The listing builds one solid part. Answer for the finished solid, in the listing's coordinates (mm). A direction names the side the tool comes from. Round coordinates to 2 decimals unless told otherwise and drop trailing zeros. Order: outer loops, then holes, each group sorted by start corner. A loop starts at its lowest first (then second) coordinate and runs counter-clockwise, first axis right, second up. Notation, with made-up numbers: (29.5, 27.25) - (49.5, 27.25) arc R16 ccw to (49.5, 57.25) - close; hole circle Ø9 at (3.25, 59). An arc over 180 degrees is marked (long way). One line per item, written item: value. Start each with the question number.
1. Section D-D, the plane y = 9 is taken. Give the vertices of the cut face in (x, z).
2. Flat-ended cylindrical pins translate along their axes: P1, Ø1, axis at x = 4.5, y = 1.5, coming from the -Z side; P2, Ø5, axis at y = 4.5, z = 3.5, coming from the -X side; P3, Ø1.8, axis at x = 3, y = -5, coming from the -Z side; P4, Ø0.9, axis at x = 4, z = 1.5, coming from the -Y side. Find the tip coordinate at first contact, or state that the pin passes through.
3. Section C-C, the plane x = 3.9 is taken. Give the vertices of the cut face in (y, z), then the cut area to 3 significant figures.
4. For a pull along Y with two mould halves and no side action, classify faces 1 (the flat face through (3, 33, 1)), 2 (the flat face through (2.96, -7.21, 6.43)), 3 (the flat face through (3, 30, 2)), 4 (the flat face through (3, 0, 2)) as released by +Y, released by -Y, zero draft, split by the parting line, or undercut.
5. Section A-A, the plane z = 1 is taken. Give the vertices of the cut face in (x, y).
6. Section B-B, the plane z = 3.5 is taken. Give the vertices of the cut face in (x, y), then the cut area to 3 significant figures.
7. A tool of negligible diameter and unlimited length cuts with its end or side. For faces 5 (the cylindrical face through (2.958, 29.699, 4.715)), 6 (the flat face through (3, -6, 3)), 7 (the flat face through (3, 31, 0)), 8 (the flat face through (3, 36, 3)), 9 (the flat face through (3, -9, 4)), from which of +Z, -Z, +X, -X, +Y, -Y can it reach the whole face along a straight path? Write none if from no direction.
8. Straight lines are drawn through the part: line 1 (Y direction, x = 1.3, z = 3.5); line 2 (Y direction, x = 2.1, z = 1); line 3 (Z direction, x = 5.75, y = 20). For each, find the intervals that lie inside material, in ascending order.
Autodesk Inventor part; units mm, degrees
ref_plane "YZ Plane" through (0, 0, 0) normal (1, 0, 0) x (0, 1, 0)
ref_plane "XZ Plane" through (0, 0, 0) normal (0, 1, 0) x (-1, 0, 0)
ref_plane "XY Plane" through (0, 0, 0) normal (0, 0, 1) x (1, 0, 0)
sketch "Sketch1" plane through (0, 0, 0) normal (1, 0, 0) x (0, 1, 0)
  line L0 (30, 0) -> (33, 0)
  line L1 (33, 0) -> (33, 3)
  line L2 (33, 3) -> (39, 3)
  line L3 (-9, 3) -> (-3, 3)
  line L4 (-3, 3) -> (-3, 0)
  line L5 (-3, 0) -> (0, 0)
  line L6 (0, 0) -> (0, 4)
  line L7 (1, 5) -> (29, 5)
  line L8 (30, 4) -> (30, 0)
  arc A0 (1, 5) -> (0, 4) centre (1, 4) ccw
  arc A1 (30, 4) -> (29, 5) centre (29, 4) ccw
  line L9 (-4, 9) -> (34, 9)
  line L10 (34, 9) -> (39, 5)
  line L11 (39, 5) -> (39, 3)
  line L12 (-9, 3) -> (-9, 5)
  line L13 (-9, 5) -> (-4, 9)
  point P0 (0, 0)
  point P1 (0, 5)
  point P2 (30, 5)
  point P3 (15, 9)
  point P4 (15, 5)
  dimension "d1" = 3
  dimension "d4" = 30
  dimension "d5" = 2
  dimension "d7" = 3
  dimension "d30" = 38
  dimension "d31" = 4
  dimension "d32" = 2
  dimension "d33" = 2
  dimension "d36" = 3
  dimension "d37" = 3
  dimension "d41" = 6
  dimension "d42" = 6
extrude "Extrusion1" add sketch "Sketch1" along normal blind 6
fillet "Fillet1" radius 5 2 edges at (3, -4, 9) (3, 34, 9)
properties part number "27080914ServoMount"
Answer list:
1. outline: (0, 5) - (6, 5) - (6, 9) - (0, 9) - close
2. P1: stops at z = 5
2. P2: stops at x = 0
2. P3: stops at z = 3
2. P4: stops at y = -3
3. outline: (-9, 3) - (-3, 3) - (-3, 0) - (0, 0) - (0, 4) arc R1 cw to (1, 5) - (29, 5) arc R1 cw to (30, 4) - (30, 0) - (33, 0) - (33, 3) - (39, 3) - (39, 5) - (35.37, 7.9) arc R5 ccw to (32.25, 9) - (-2.25, 9) arc R5 ccw to (-5.37, 7.9) - (-9, 5) - close
3. area: 226 mm²
4. face 1: released by +Y
4. face 2: released by -Y
4. face 3: undercut
4. face 4: undercut
5. outline: (0, -3) - (6, -3) - (6, 0) - (0, 0) - close; (0, 30) - (6, 30) - (6, 33) - (0, 33) - close
6. outline: (0, -9) - (6, -9) - (6, 0) - (0, 0) - close; (0, 30) - (6, 30) - (6, 39) - (0, 39) - close
6. area: 108 mm²
7. face 5: -Z, +X, -X
7. face 6: -Z, +X, -X, -Y
7. face 7: -Z, +X, -X, +Y, -Y
7. face 8: -Z, +X, -X, +Y
7. face 9: +Z, -Z, +X, -X, -Y
8. line 1: y = -9 to 0, 30 to 39
8. line 2: y = -3 to 0, 30 to 33
8. line 3: z = 5 to 9
